```python
from build123d import *

# Parameters (mm, degrees)
SKETCH1_R           = 4
BOSS_EXTRUDE1_DEPTH = 1.5
SKETCH2_R           = 3
BOSS_EXTRUDE2_DEPTH = 3
SKETCH3_R           = 4
BOSS_EXTRUDE3_DEPTH = 1.5
FILLET1_R           = 1
SKETCH4_R           = 1.8
CUT_EXTRUDE1_DEPTH  = 9.246211251


with BuildPart() as part:
    # Sketch1 → Boss-Extrude1 (new body)
    with BuildSketch(Plane(origin=(0, 0, 0), x_dir=(0, 0, -1), z_dir=(1, 0, 0))):
        Circle(SKETCH1_R)
    extrude(amount=BOSS_EXTRUDE1_DEPTH)

    # Sketch2 → Boss-Extrude2 (add)
    with BuildSketch(Plane(origin=(1.5, 0, 0), x_dir=(0, 0, -1), z_dir=(1, 0, 0))):
        Circle(SKETCH2_R)
    extrude(amount=BOSS_EXTRUDE2_DEPTH)

    # Sketch3 → Boss-Extrude3 (add)
    with BuildSketch(Plane(origin=(4.5, 0, 0), x_dir=(0, 0, -1), z_dir=(1, 0, 0))):
        Circle(SKETCH3_R)
    extrude(amount=BOSS_EXTRUDE3_DEPTH)

    # Fillet1
    fillet1_edges = [part.edges().sort_by_distance(p)[0] for p in [
        (1.5, 0, 3),
        (4.5, 0, 3),
    ]]
    fillet(fillet1_edges, radius=FILLET1_R - 0.0001)  # a hair under: the kernel refuses the full size

    # Sketch4 → Cut-Extrude1 (cut, through all)
    with BuildSketch(Plane.ZY):
        Circle(SKETCH4_R)
    extrude(amount=-CUT_EXTRUDE1_DEPTH, mode=Mode.SUBTRACT)


solid = part.part
```
Check sheet for the modelled part. Datum: model origin and axes. Units: mm. A direction names the side the tool comes from. Round coordinates to 2 decimals unless told otherwise and drop trailing zeros. Loops run counter-clockwise (first coordinate to the right, second up) from the corner with the lowest first, then second, coordinate; pieces in that order, holes last. Notation, with made-up numbers: (-32.75, -13.75) - (23.25, -13.75) arc R24 cw to (23.25, 6.25) - close; hole circle Ø1 at (54, 50.5). An arc over 180 degrees is marked (long way). Write item = value, one per line. Start each with the question number.
Q1. Depth check by flat-ended pin: P1, Ø1.5, axis at y = 0, z = -0.5, coming from the -X side. Enter the tip coordinate at first touch or a pass-through.
Q2. Access from +Z, -Z, +X, -X, +Y, -Y to the whole of each face (thin tool, end or side, straight path). Record for faces 1 (the face through (0, -1, -2)), 2 (the face through (3, 0, 3)).
Q3. Thickness scan on L1, parallel to Y at x = 3.2, z = 0; L2, parallel to Y at x = 4.25, z = 0; L3, parallel to X at y = 3, z = 1. Record the ranges inside material, lowest first.
Q4. Section check D-D (x = 3). Record the boundary of the cut face in (y, z).
Q5. Release check for a two-part mould opening along Z. For faces 3 (the face through (5.24, -3.905, 0.867)), 4 (the face through (6, -1, -2)), 5 (the face through (2.958, 0.541, 1.717)) record: pulls with the +Z half, pulls with the -Z half, needs draft (parallel to the pull), parting line crosses it, or undercut.
Q6. Section check C-C (x = 4.7). Record the boundary of the cut face in (y, z), plus the area to 3 significant figures.
Derived:
q1.P1 = through
q2.face_1 = +Z, -Z, -X, +Y, -Y
q2.face_2 = none
q3.L1 = -3 to -1.8, 1.8 to 3
q3.L2 = -3.34 to -1.8, 1.8 to 3.34
q3.L3 = 0 to 1.95, 4.05 to 6
q4.outline = circle Ø6 at (0, 0); hole circle Ø3.6 at (0, 0)
q5.face_3 = parting line crosses it
q5.face_4 = needs draft
q5.face_5 = undercut
q6.outline = circle Ø8 at (0, 0); hole circle Ø3.6 at (0, 0)
q6.area = 40.1 mm^2
